from build123d import *

# Parameters (mm, degrees)
F0_W     = 700
F0_H     = 72
F1_DEPTH = 18
F2_W     = 72
F2_H     = 72
F3_DEPTH = 11.65


with BuildPart() as f1:
    # F0 (on Front) → F1 (new body, symmetric)
    with BuildSketch(Plane.XZ):
        Rectangle(F0_W, F0_H)
    extrude(amount=F1_DEPTH, both=True)

    # F2 (on face) → F3 (cut)
    with BuildSketch(Plane.XZ.offset(18)):
        with Locations((-314, 0)):
            Rectangle(F2_W, F2_H)
        with Locations((314, 0)):
            Rectangle(F2_W, F2_H)
    extrude(amount=-F3_DEPTH, mode=Mode.SUBTRACT)


solid = f1.part
For this review, take the finished solid that the model builds, in its own axes (mm). A direction names the side the tool comes from. Round coordinates to 2 decimals unless told otherwise and drop trailing zeros. Loops run counter-clockwise (first coordinate to the right, second up) from the corner with the lowest first, then second, coordinate; pieces in that order, holes last. Notation, with made-up numbers: (85.25, 57.25) - (124.25, 57.25) arc R32 ccw to (124.25, 96.25) - close; hole circle Ø10 at (61, -25). An arc over 180 degrees is marked (long way). One line per item, written item: value. Start each with the question number.
Item 1: For L1, parallel to X at y = -14, z = 28.5; L2, parallel to Y at x = -312, z = 11, list the stretches that pass through material, from the lowest coordinate up.
Item 2: Clearance check with flat-ended pins moving along their axes: pin 1 Ø13 at (y, z) = (-15, -4) entering from -X; pin 2 Ø9.5 at (y, z) = (-12.5, -8.5) entering from +X; pin 3 Ø21.5 at (x, z) = (-310, 4.5) entering from -Y. State where each tip first meets the part, or that it passes through.
Item 3: For faces 1 (the flat face through (-315, -6.35, 1)), 2 (the flat face through (313, -6.35, 1)), 3 (the flat face through (-350, 6, -1)), list the 3-axis set-ups (+Z, -Z, +X, -X, +Y, -Y) from which the entire face can be reached by the end or side of a thin tool; tool diameter is ignored.
Item 4: Take a section at B-B (x = -286). Give the boundary of the cut face in (y, z), plus the area to 3 significant figures.
Item 5: Take a section at A-A (z = 7). Give the boundary of the cut face in (x, y).
Answer below:
1. L1: x = -278 to 278
1. L2: y = -6.35 to 18
2. pin 1: stops at x = -278
2. pin 2: stops at x = 278
2. pin 3: stops at y = -6.35
3. face 1: +Z, -Z, -X, -Y
3. face 2: +Z, -Z, +X, -Y
3. face 3: +Z, -Z, -X, +Y, -Y
4. outline: (-6.35, -36) - (18, -36) - (18, 36) - (-6.35, 36) - close
4. area: 1,750 mm2
5. outline: (-350, -6.35) - (-278, -6.35) - (-278, -18) - (278, -18) - (278, -6.35) - (350, -6.35) - (350, 18) - (-350, 18) - close
